from build123d import *

# Parameters (mm, degrees)
BOX014_W               = 16
BOX014_H               = 4
BOX014_DEPTH           = 16
BOX014_PLACEMENT_ANGLE = 15
CYLINDER039_R          = 0.5
CYLINDER039_DEPTH      = 20
CYLINDER038_R          = 0.5
CYLINDER038_DEPTH      = 20
CYLINDER034_R          = 0.5
CYLINDER034_DEPTH      = 20
CYLINDER035_R          = 0.5
CYLINDER035_DEPTH      = 20
CYLINDER040_R          = 0.5
CYLINDER040_DEPTH      = 20
CYLINDER036_R          = 0.5
CYLINDER036_DEPTH      = 20
CYLINDER037_R          = 0.5
CYLINDER037_DEPTH      = 20
CYLINDER033_R          = 0.5
CYLINDER033_DEPTH      = 20
CYLINDER030_R          = 6
CYLINDER030_DEPTH      = 14
BOX013_W               = 9
BOX013_H               = 10
BOX013_DEPTH           = 5
CYLINDER031_R          = 8
CYLINDER031_DEPTH      = 6
CYLINDER032_R          = 12
CYLINDER032_DEPTH      = 2


with BuildPart() as cube014:
    # Box014 → Box014 (new body)
    with BuildSketch(Plane.XY):
        with Locations((8, 2)):
            Rectangle(BOX014_W, BOX014_H)
    extrude(amount=BOX014_DEPTH)


with BuildPart() as cube014_1:
    # Box014 placement: moved
    add(cube014.part.moved(Location((19, -17, 13))).rotate(Axis((19, -17, 13), (0, 0, 1)), BOX014_PLACEMENT_ANGLE))


with BuildPart() as cylinder039:
    # Cylinder039 → Cylinder039 (new body)
    with BuildSketch(Plane(origin=(32, 7, 14), x_dir=(1, 0, 0), z_dir=(0, -1, 0))):
        Circle(CYLINDER039_R)
    extrude(amount=CYLINDER039_DEPTH)


with BuildPart() as cylinder038:
    # Cylinder038 → Cylinder038 (new body)
    with BuildSketch(Plane(origin=(18, 7, 14), x_dir=(1, 0, 0), z_dir=(0, -1, 0))):
        Circle(CYLINDER038_R)
    extrude(amount=CYLINDER038_DEPTH)


with BuildPart() as cylinder034:
    # Cylinder034 → Cylinder034 (new body)
    with BuildSketch(Plane(origin=(35, 7, 21), x_dir=(1, 0, 0), z_dir=(0, -1, 0))):
        Circle(CYLINDER034_R)
    extrude(amount=CYLINDER034_DEPTH)


with BuildPart() as cylinder035:
    # Cylinder035 → Cylinder035 (new body)
    with BuildSketch(Plane(origin=(25, 7, 11), x_dir=(1, 0, 0), z_dir=(0, -1, 0))):
        Circle(CYLINDER035_R)
    extrude(amount=CYLINDER035_DEPTH)


with BuildPart() as cylinder040:
    # Cylinder040 → Cylinder040 (new body)
    with BuildSketch(Plane(origin=(18, 7, 28), x_dir=(1, 0, 0), z_dir=(0, -1, 0))):
        Circle(CYLINDER040_R)
    extrude(amount=CYLINDER040_DEPTH)


with BuildPart() as cylinder036:
    # Cylinder036 → Cylinder036 (new body)
    with BuildSketch(Plane(origin=(25, 7, 31), x_dir=(1, 0, 0), z_dir=(0, -1, 0))):
        Circle(CYLINDER036_R)
    extrude(amount=CYLINDER036_DEPTH)


with BuildPart() as cylinder037:
    # Cylinder037 → Cylinder037 (new body)
    with BuildSketch(Plane(origin=(32, 7, 28), x_dir=(1, 0, 0), z_dir=(0, -1, 0))):
        Circle(CYLINDER037_R)
    extrude(amount=CYLINDER037_DEPTH)


with BuildPart() as fusion033:
    # Cylinder033 → Cylinder033 (new body)
    with BuildSketch(Plane(origin=(15, 7, 21), x_dir=(1, 0, 0), z_dir=(0, -1, 0))):
        Circle(CYLINDER033_R)
    extrude(amount=CYLINDER033_DEPTH)

    # Fusion033: union Cylinder039, Cylinder038, Cylinder034, Cylinder035, Cylinder040, Cylinder036, Cylinder037
    add(cylinder039.part)
    add(cylinder038.part)
    add(cylinder034.part)
    add(cylinder035.part)
    add(cylinder040.part)
    add(cylinder036.part)
    add(cylinder037.part)


with BuildPart() as cylinder030:
    # Cylinder030 → Cylinder030 (new body)
    with BuildSketch(Plane(origin=(25, -8, 21), x_dir=(1, 0, 0), z_dir=(0, 1, 0))):
        Circle(CYLINDER030_R)
    extrude(amount=CYLINDER030_DEPTH)


with BuildPart() as fusion032:
    # Box013 → Box013 (new body)
    with BuildSketch(Plane(origin=(22, -13, 18.5), x_dir=(1, 0, 0), z_dir=(0, 0, 1))):
        with Locations((4.5, 5)):
            Rectangle(BOX013_W, BOX013_H)
    extrude(amount=BOX013_DEPTH)

    # Fusion032: union Cylinder030
    add(cylinder030.part)


with BuildPart() as cylinder031:
    # Cylinder031 → Cylinder031 (new body)
    with BuildSketch(Plane(origin=(25, -11, 21), x_dir=(1, 0, 0), z_dir=(0, 1, 0))):
        Circle(CYLINDER031_R)
    extrude(amount=CYLINDER031_DEPTH)


with BuildPart() as springflange001:
    # Cylinder032 → Cylinder032 (new body)
    with BuildSketch(Plane(origin=(25, -7, 21), x_dir=(1, 0, 0), z_dir=(0, 1, 0))):
        Circle(CYLINDER032_R)
    extrude(amount=CYLINDER032_DEPTH)

    # Fusion034: union Cylinder031
    add(cylinder031.part)

    # Cut022: cut Fusion032
    add(fusion032.part, mode=Mode.SUBTRACT)

    # Cut023: cut Fusion033
    add(fusion033.part, mode=Mode.SUBTRACT)

    # Cut030: cut Cube014
    add(cube014_1.part, mode=Mode.SUBTRACT)


solid = springflange001.part
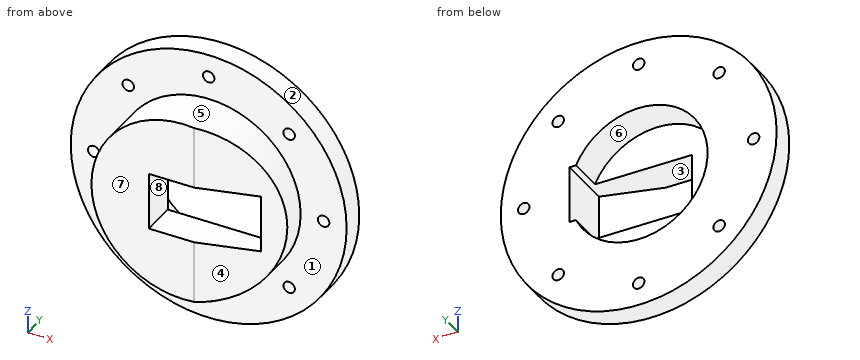
Design review of the part built by this model. Coordinates are the model's own, in mm. Face numbers are marked on the shaded views. A direction names the side the tool comes from. Round coordinates to 2 decimals unless told otherwise and drop trailing zeros. Loops run counter-clockwise (first coordinate to the right, second up) from the corner with the lowest first, then second, coordinate; pieces in that order, holes last. Notation, with made-up numbers: (-14, 61.25) - (45, 61.25) arc R19 ccw to (45, 72.25) - close; hole circle Ø9 at (-1, 41). An arc over 180 degrees is marked (long way). One line per item, written item: value. Start each with the question number.
1) Insertion check: pin 1 Ø1 at (x, y) = (31.5, -9) entering from -Z; pin 2 Ø3.5 at (x, z) = (26, 18.5) entering from +Y; pin 3 Ø3.5 at (y, z) = (-9, 20.5) entering from +X. Each pin has a flat end and moves straight along its axis. Give the tip position at first contact, or say it passes through.
2) Consider section B-B on y = -8.75. Give the boundary of the cut face in (x, z), then the cut area to 3 significant figures.
3) For the marked faces 4, 5, 6, 7 and 8, list the 3-axis set-ups (+Z, -Z, +X, -X, +Y, -Y) from which the entire face can be reached by the end or side of a thin tool; tool diameter is ignored.
4) To check wall thickness, follow L1, parallel to Z at x = 25, y = -6.05; L2, parallel to X at y = -6.5, z = 21; L3, parallel to X at y = -6.4, z = 28. State the ranges of each line that lie inside material, in increasing order. Write a range as from..to.
5) Consider section D-D on x = 15. Give the boundary of the cut face in (y, z), then the cut area to 3 significant figures.
6) Consider section A-A on x = 25. Give the boundary of the cut face in (y, z).
7) Draft analysis for pull direction X (two halves, no side actions). For the marked faces 1, 2 and 3, state which applies: +X half, -X half, draft (parallel to the pull), parting line (faces both ways), or undercut.
8) Consider section C-C on z = 21. Give the boundary of the cut face in (x, y).
Reported:
1. pin 1: stops at z = 15.71
1. pin 2: stops at y = -8
1. pin 3: stops at x = 33
2. outline: circle Ø16 at (25, 21); hole (22, 18.5) - (31, 18.5) - (31, 23.5) - (22, 23.5) - close
2. area: 156 mm^2
3. face 4: +Z, -Z, +X, -Y
3. face 5: -Y
3. face 6: +Y
3. face 7: +Z, -Z, +X, -X, -Y
3. face 8: +Y, -Y
4. L1: z = 9..10.5, 11.5..15, 27..30.5, 31.5..33
4. L2: x = 13..14.5, 15.5..19, 31..34.5, 35.5..37
4. L3: x = 15.25..17.5, 18.5..31.5, 32.5..34.75
5. outline: (-7, 14.37) - (-5, 14.37) - (-5, 20.5) - (-7, 20.5) - close; (-7, 21.5) - (-5, 21.5) - (-5, 27.63) - (-7, 27.63) - close
5. area: 24.5 mm^2
6. outline: (-11, 13) - (-7, 13) - (-7, 11.5) - (-5, 11.5) - (-5, 15) - (-8, 15) - (-8, 18.5) - (-11, 18.5) - close; (-11, 23.5) - (-8, 23.5) - (-8, 27) - (-5, 27) - (-5, 30.5) - (-7, 30.5) - (-7, 29) - (-11, 29) - close; (-7, 9) - (-5, 9) - (-5, 10.5) - (-7, 10.5) - close; (-7, 31.5) - (-5, 31.5) - (-5, 33) - (-7, 33) - close
7. face 1: draft
7. face 2: parting line
7. face 3: undercut
8. outline: (13, -7) - (14.5, -7) - (14.5, -5) - (13, -5) - close; (15.5, -7) - (17, -7) - (17, -11) - (22, -11) - (22, -8) - (19, -8) - (19, -5) - (15.5, -5) - close; (31, -9.64) - (33, -9.11) - (33, -7) - (34.5, -7) - (34.5, -5) - (31, -5) - close; (35.5, -7) - (37, -7) - (37, -5) - (35.5, -5) - close
